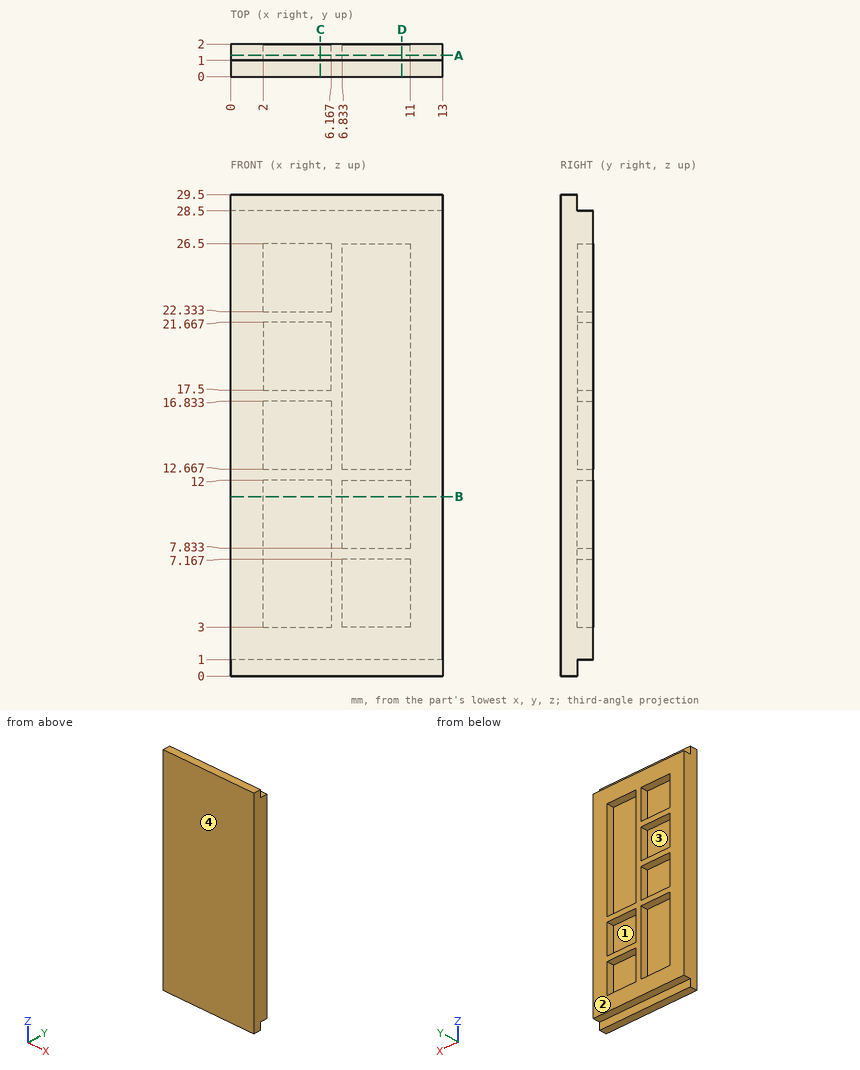
Study the drawing (mm; zero at the part's minimum x, y, z) and answer. A direction names the side the tool comes from. Round coordinates to 2 decimals unless told otherwise and drop trailing zeros. Write each loop counter-clockwise with the first axis right and the second up, starting at its lowest first coordinate (ties: lowest second). Pieces come first, ordered by that corner, then holes. Notation, with made-up numbers: (56, 7.5) -> (99, 7.5) arc R18 ccw to (99, 33.5) -> close; hole circle Ø3 at (4, 86.25). An arc over 180 degrees is marked (long way). Answer as CSV lines item,"result". Start each with the question number.
(1) The part is cut by section D-D, the plane x = 10.5. Give the vertices of the cut face in (y, z).
(2) Each of these flat-tipped pins is pushed along its axis until it touches: pin 1 (0.8 mm diameter, centred on x = 3, y = 1.5, fed in from +Z); pin 2 (0.5 mm diameter, centred on x = 5, y = 1.5, fed in from -Z). Where does it stop, or does it pass through?
(3) The part is cut by section A-A, the plane y = 1.3. Give the number of separate pieces and of enclosed holes in the cut face.
(4) The part is cut by section C-C, the plane x = 5.5. Give the vertices of the cut face in (y, z), then the cut area to 3 significant figures.
(5) Find the intervals of material crossed by probe 1 along Z at (x, y) = (8.25, 1.15); probe 2 along X at (y, z) = (1.05, 11.5); probe 3 along Z at (x, y) = (6, 1.6), in increasing order.
(6) A tool of negligible diameter and unlimited length cuts with its end or side. For the marked faces 1 and 2, from which of +Z, -Z, +X, -X, +Y, -Y can it reach the whole face along a straight path? Write none if from no direction.
(7) The mould has two halves that part along X. Classify the marked faces 3 and 4: +X half, -X half, draft (parallel to the pull), parting line (faces both ways), or undercut.
(8) The part is cut by section B-B, the plane z = 11. Give the vertices of the cut face in (x, y).
Output values:
1,outline,"(0, 0) -> (1, 0) -> (1, 1) -> (2, 1) -> (2, 3) -> (1, 3) -> (1, 7.17) -> (2, 7.17) -> (2, 7.83) -> (1, 7.83) -> (1, 12) -> (2, 12) -> (2, 12.67) -> (1, 12.67) -> (1, 26.5) -> (2, 26.5) -> (2, 28.5) -> (1, 28.5) -> (1, 29.5) -> (0, 29.5) -> close"
2,pin 1,"stops at z = 28.5"
2,pin 2,"stops at z = 1"
3,separate pieces,"1"
3,enclosed holes,"7"
4,outline,"(0, 0) -> (1, 0) -> (1, 1) -> (2, 1) -> (2, 3) -> (1, 3) -> (1, 12) -> (2, 12) -> (2, 12.67) -> (1, 12.67) -> (1, 16.83) -> (2, 16.83) -> (2, 17.5) -> (1, 17.5) -> (1, 21.67) -> (2, 21.67) -> (2, 22.33) -> (1, 22.33) -> (1, 26.5) -> (2, 26.5) -> (2, 28.5) -> (1, 28.5) -> (1, 29.5) -> (0, 29.5) -> close"
4,area,"35.5 mm²"
5,probe 1,"z = 1 to 3, 7.17 to 7.83, 12 to 12.67, 26.5 to 28.5"
5,probe 2,"x = 0 to 2, 6.17 to 6.83, 11 to 13"
5,probe 3,"z = 1 to 3, 12 to 12.67, 16.83 to 17.5, 21.67 to 22.33, 26.5 to 28.5"
6,face 1,"+Y"
6,face 2,"+Z, -Z, +X, -X, +Y"
7,face 3,"undercut"
7,face 4,"draft"
8,outline,"(0, 0) -> (13, 0) -> (13, 2) -> (11, 2) -> (11, 1) -> (6.83, 1) -> (6.83, 2) -> (6.17, 2) -> (6.17, 1) -> (2, 1) -> (2, 2) -> (0, 2) -> close"
